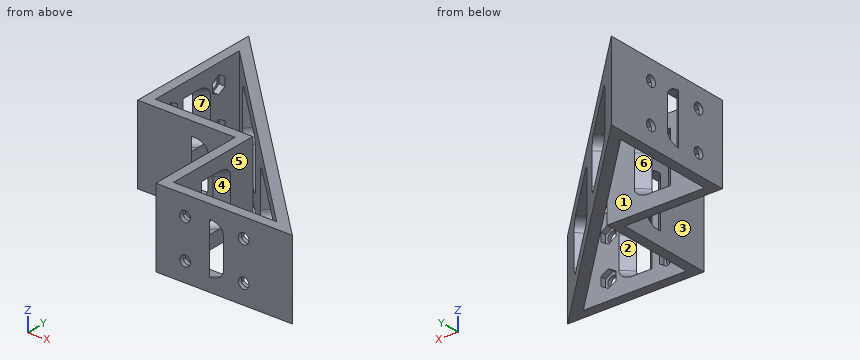
```python
from build123d import *

# Parameters (mm, degrees)
F1_DEPTH  = 40
F2_T      = -5
F4_DEPTH  = 30
F5_R      = 2.75
F6_DEPTH  = 5
F7_R      = 2.75
F8_DEPTH  = 5
F9_R      = 2.75
F10_DEPTH = 3
F11_R     = 2.75
F12_DEPTH = 3


# Not quite as in the source:
# - a feature names something its author has since deleted; it is built from what else it names


with BuildPart() as f1:
    # F0 (on Top) → F1 (new body)
    with BuildSketch(Plane.XY):
        Polygon((120, 0), (0, 120), (0, 100), (50, 50), (100, 0), align=None)
        Polygon((50, 50), (0, 100), (0, 92.9289321881), (42.9289321881, 50), align=None)
        Polygon((42.9289321881, 50), (0, 92.9289321881), (0, 50), align=None)
        Polygon((92.9289321881, 0), (50, 42.9289321881), (50, 0), align=None)
        Polygon((100, 0), (50, 50), (50, 42.9289321881), (92.9289321881, 0), align=None)
    extrude(amount=F1_DEPTH)

    # F2
    f2_openings = [f1.faces().sort_by_distance(p)[0] for p in [
        (51.697056, 25, 40),
        (51.697056, 25, 0),
    ]]
    offset(amount=F2_T, openings=f2_openings, kind=Kind.INTERSECTION)

    # F3 (on face) → F4 (cut)
    with BuildSketch(Plane(origin=(60, 60, 0), x_dir=(-0.7071067812, 0.7071067812, 0), z_dir=(0.7071067812, 0.7071067812, 0))):
        with BuildLine():
            ThreePointArc((59.8528137424, 28), (58.3883476483, 31.5355339059), (54.8528137424, 33))
            Line((54.8528137424, 33), (14.8528137424, 33))
            ThreePointArc((14.8528137424, 33), (11.3172798365, 31.5355339059), (9.8528137424, 28))
            Line((9.8528137424, 28), (9.8528137424, 12))
            ThreePointArc((9.8528137424, 12), (11.3172798365, 8.4644660941), (14.8528137424, 7))
            Line((14.8528137424, 7), (54.8528137424, 7))
            ThreePointArc((54.8528137424, 7), (58.3883476483, 8.4644660941), (59.8528137424, 12))
            Line((59.8528137424, 12), (59.8528137424, 28))
        make_face()
        with BuildLine():
            ThreePointArc((-54.8528137424, 33), (-58.3883476483, 31.5355339059), (-59.8528137424, 28))
            Line((-59.8528137424, 28), (-59.8528137424, 12))
            ThreePointArc((-59.8528137424, 12), (-58.3883476483, 8.4644660941), (-54.8528137424, 7))
            Line((-54.8528137424, 7), (-14.8528137424, 7))
            ThreePointArc((-14.8528137424, 7), (-11.3172798365, 8.4644660941), (-9.8528137424, 12))
            Line((-9.8528137424, 12), (-9.8528137424, 28))
            ThreePointArc((-9.8528137424, 28), (-11.3172798365, 31.5355339059), (-14.8528137424, 33))
            Line((-14.8528137424, 33), (-54.8528137424, 33))
        make_face()
    extrude(amount=-F4_DEPTH, mode=Mode.SUBTRACT)

    # F5 (on face) → F6 (cut, through all)
    with BuildSketch(Plane(origin=(0, 0, 0), x_dir=(0, -1, 0), z_dir=(-1, 0, 0))):
        with Locations((-95, 10)):
            Circle(F5_R)
        with Locations((-95, 30)):
            Circle(F5_R)
        with Locations((-65, 10)):
            Circle(F5_R)
        with Locations((-65, 30)):
            Circle(F5_R)
    extrude(amount=-F6_DEPTH, mode=Mode.SUBTRACT)

    # F7 (on face) → F8 (cut, through all)
    with BuildSketch(Plane.XZ):
        with Locations((65, 30)):
            Circle(F7_R)
        with Locations((95, 30)):
            Circle(F7_R)
        with Locations((95, 10)):
            Circle(F7_R)
        with Locations((65, 10)):
            Circle(F7_R)
    extrude(amount=-F8_DEPTH, mode=Mode.SUBTRACT)

    # F9 (on face) → F10 (cut)
    with BuildSketch(Plane.YZ.offset(5)):
        Polygon((61.15, 27.7772014636), (65, 25.5544029272), (68.85, 27.7772014636), (68.85, 32.2227985364), (65, 34.4455970728), (61.15, 32.2227985364), align=None)
        with Locations((65, 30)):
            Circle(F9_R, mode=Mode.SUBTRACT)
        Polygon((61.15, 12.2227985364), (61.15, 7.7772014636), (65, 5.5544029272), (68.85, 7.7772014636), (68.85, 12.2227985364), (65, 14.4455970728), align=None)
        with Locations((65, 10)):
            Circle(F9_R, mode=Mode.SUBTRACT)
        Polygon((91.15, 7.7772014636), (95, 5.5544029272), (98.85, 7.7772014636), (98.85, 12.2227985364), (95, 14.4455970728), (91.15, 12.2227985364), align=None)
        with Locations((95, 10)):
            Circle(F9_R, mode=Mode.SUBTRACT)
        Polygon((91.15, 27.7772014636), (95, 25.5544029272), (98.85, 27.7772014636), (98.85, 32.2227985364), (95, 34.4455970728), (91.15, 32.2227985364), align=None)
        with Locations((95, 30)):
            Circle(F9_R, mode=Mode.SUBTRACT)
    extrude(amount=-F10_DEPTH, mode=Mode.SUBTRACT)

    # F11 (on face) → F12 (cut)
    with BuildSketch(Plane(origin=(0, 5, 0), x_dir=(-1, 0, 0), z_dir=(0, 1, 0))):
        Polygon((-91.15, 12.2227985364), (-95, 14.4455970728), (-98.85, 12.2227985364), (-98.85, 7.7772014636), (-95, 5.5544029272), (-91.15, 7.7772014636), align=None)
        with Locations((-95, 10)):
            Circle(F11_R, mode=Mode.SUBTRACT)
        Polygon((-91.15, 32.2227985364), (-95, 34.4455970728), (-98.85, 32.2227985364), (-98.85, 27.7772014636), (-95, 25.5544029272), (-91.15, 27.7772014636), align=None)
        with Locations((-95, 30)):
            Circle(F11_R, mode=Mode.SUBTRACT)
        Polygon((-61.15, 32.2227985364), (-65, 34.4455970728), (-68.85, 32.2227985364), (-68.85, 27.7772014636), (-65, 25.5544029272), (-61.15, 27.7772014636), align=None)
        with Locations((-65, 30)):
            Circle(F11_R, mode=Mode.SUBTRACT)
        Polygon((-61.15, 12.2227985364), (-65, 14.4455970728), (-68.85, 12.2227985364), (-68.85, 7.7772014636), (-65, 5.5544029272), (-61.15, 7.7772014636), align=None)
        with Locations((-65, 10)):
            Circle(F11_R, mode=Mode.SUBTRACT)
    extrude(amount=-F12_DEPTH, mode=Mode.SUBTRACT)


solid = f1.part
```
Here's how the part is built. I have some questions about the finished solid (model axes, mm). Face numbers are marked on the shaded views. A direction names the side the tool comes from. Give positions to 0.01 mm unless a question says otherwise; leave off trailing zeros. Loops run counter-clockwise (first coordinate to the right, second up) from the corner with the lowest first, then second, coordinate; pieces in that order, holes last. Notation, with made-up numbers: M 82,-40 L 135,-40 A32 cw 135,-6 Z; hole C 50,49.5 d8. An arc over 180 degrees is marked long. Put each result on its own line as item: value. Start each with the question number.
(1) Will these pins go through, and if not, where does the flat tip stop? pin 1 Ø0.9 at (y, z) = (3.5, 11) entering from +X; pin 2 Ø2.5 at (y, z) = (4, 9) entering from -X; pin 3 Ø2.5 at (x, z) = (3, 11) entering from +Y.
(2) I want a section at C-C on x = 11. Please give me the cut outline in (y, z).
(3) I need wall thicknesses on line 1 along Z through (x, y) = (95, 1.25); line 2 along X through (y, z) = (1.3, 30); line 3 along X through (y, z) = (15, 30). Which ranges of each line are inside material? Lowest first, please. Write a range as [from, to].
(4) For the marked faces 1, 2, 3 and 4, which set-ups out of +Z, -Z, +X, -X, +Y, -Y let a thin tool reach every point of the face, with its end or its side?
(5) I want a section at B-B on y = 44.5. Please give me the cut outline in (x, z).
(6) If we mould it in two halves opening along Z, with no side actions, what happens to the marked faces 5, 6 and 7? For each: +Z half, -Z half, draft (parallel to the pull), parting line (faces both ways), or undercut.
(7) I want a section at A-A on z = 17. State how many separate pieces and enclosed holes the cut face has, then the cut area to 3 significant figures.
Answer block:
1. pin 1: x = 116.95
1. pin 2: x = 50
1. pin 3: y = 118.25
2. outline: M 50,0 L 55,0 L 55,40 L 50,40 Z; M 101.93,0 L 109,0 L 109,40 L 101.93,40 Z
3. line 1: [0, 7.25], [12.75, 27.25], [32.75, 40]
3. line 2: [50, 62.25], [67.75, 76.27], [85.35, 92.25], [97.75, 118.7]
3. line 3: [50, 55], [99.05, 105]
4. face 1: +Z, -Z
4. face 2: +Y
4. face 3: +Z, -Z, -X, -Y
4. face 4: +X
5. outline: M 50,0 L 55,0 L 55,40 L 50,40 Z; M 68.43,0 L 75.5,0 L 75.5,7 L 68.43,7 Z; M 68.43,33 L 75.5,33 L 75.5,40 L 68.43,40 Z
6. face 5: draft
6. face 6: undercut
6. face 7: undercut
7. separate pieces: 6
7. enclosed holes: 0
7. area: 1,150 mm^2
